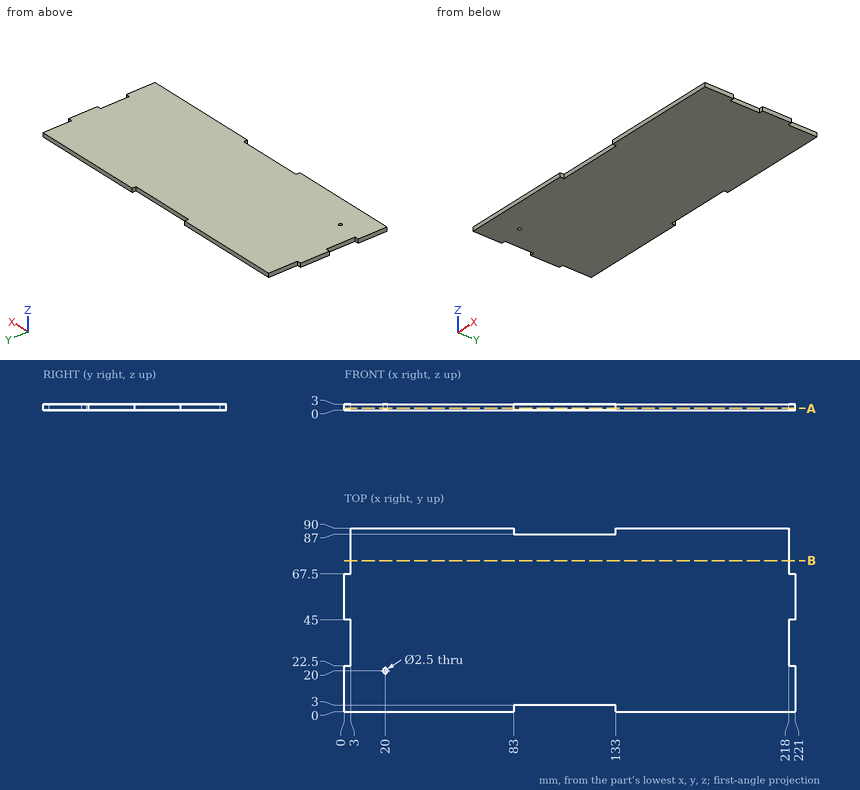
The drawing under review shows one solid part. Ordinate dimensions are in mm from its lowest x, y, z. Round coordinates to 2 decimals unless told otherwise and drop trailing zeros. Loops run counter-clockwise (first coordinate to the right, second up) from the corner with the lowest first, then second, coordinate; pieces in that order, holes last. Notation, with made-up numbers: (20, 70) - (67, 70) arc R13 cw to (67, 94) - close; hole circle Ø6 at (54.5, 30). An arc over 180 degrees is marked (long way). One line per question, with ' | ' between items.
1. We need section A-A, the plane z = 0.8. State the section outline as (x, y) points, and give its area (3 significant figures).
Results are:
outline: (0, 0) - (83, 0) - (83, 3) - (133, 3) - (133, 0) - (221, 0) - (221, 22.5) - (218, 22.5) - (218, 45) - (221, 45) - (221, 67.5) - (218, 67.5) - (218, 90) - (133, 90) - (133, 87) - (83, 87) - (83, 90) - (3, 90) - (3, 67.5) - (0, 67.5) - (0, 45) - (3, 45) - (3, 22.5) - (0, 22.5) - close; hole circle Ø2.5 at (20, 20) | area: 19,300 mm²
2. For L1, parallel to Y at x = 20, z = 1.35; L2, parallel to X at y = 71, z = 2.2; L3, parallel to Y at x = 88, z = 1.4, list the stretches that pass through material, from the lowest coordinate up. Write a range as [from, to].
Results are:
L1: y = [0, 18.75], [21.25, 90] | L2: x = [3, 218] | L3: y = [3, 87]
3. Clearance check with flat-ended pins moving along their axes: P1, Ø0.9, axis at y = 89, z = 2, coming from the +X side; P2, Ø1.5, axis at x = 101.5, z = 2.5, coming from the +Y side; P3, Ø0.9, axis at x = 2, z = 1, coming from the +Y side. State where each tip first meets the part, or that it passes through.
Results are:
P1: stops at x = 218 | P2: stops at y = 87 | P3: stops at y = 67.5
4. We need section B-B, the plane y = 74. State the section outline as (x, z) points, and give its area (3 significant figures).
Results are:
outline: (3, 0) - (218, 0) - (218, 3) - (3, 3) - close | area: 645 mm²
